```python
from build123d import *

# Parameters (mm, degrees)
SKETCH_1_R          = 0.9
EXTRUDE_1_DEPTH     = 1.8
SKETCH_2_R          = 1.5
EXTRUDE_2_DEPTH     = 1.5
SKETCH_2_3_W        = 1.1
SKETCH_2_3_H        = 0.4
CUT_EXTRUDE_1_DEPTH = 11.647300127


with BuildPart() as part:
    # Sketch 1 → Extrude 1 (new body)
    with BuildSketch(Plane.XY):
        with BuildLine():
            Line((-2.839013913, -0.25), (-6.05, -0.25))
            Line((-6.05, -0.25), (-6.05, -1.65))
            Line((-6.05, -1.65), (-7.95, -1.65))
            Line((-7.95, -1.65), (-7.95, -3.35))
            Line((-7.95, -3.35), (-6.05, -3.35))
            Line((-6.05, -3.35), (-6.05, -5.95))
            ThreePointArc((-6.05, -5.95), (-5.15, -5.05), (-4.25, -5.95))
            ThreePointArc((-4.25, -5.95), (-4.513603897, -6.586396103), (-5.15, -6.85))
            Line((-5.15, -6.85), (4.65, -6.85))
            Line((4.65, -6.85), (4.65, -5.95))
            Line((4.65, -5.95), (6.55, -5.95))
            Line((6.55, -5.95), (6.55, -4.25))
            Line((6.55, -4.25), (4.65, -4.25))
            Line((4.65, -4.25), (4.65, -2.85))
            Line((4.65, -2.85), (0, -2.85))
            ThreePointArc((0, -2.85), (-1.924837655, -2.101784956), (-2.839013913, -0.25))
        make_face()
        with Locations((-5.15, -5.95)):
            Circle(SKETCH_1_R)
    extrude(amount=EXTRUDE_1_DEPTH)

    # Sketch 2 → Extrude 2 (add)
    with BuildSketch(Plane(origin=(0, 0, 0), x_dir=(-1, 0, 0), z_dir=(0, 0, -1))):
        with Locations(Location((-2.54, -5.01, 0), (0, 0, 180))):
            Circle(SKETCH_2_R)
        with Locations(Location((3.81, -2.54, 0), (0, 0, 180))):
            Circle(SKETCH_2_R)
    extrude(amount=EXTRUDE_2_DEPTH)

    # Sketch 2_3 → Cut-Extrude 1 (cut, through all)
    with BuildSketch(Plane(origin=(0, 0, 0), x_dir=(-1, 0, 0), z_dir=(0, 0, -1))):
        with Locations((-2.54, -5.01)):
            Rectangle(SKETCH_2_3_W, SKETCH_2_3_H)
        with Locations((3.81, -2.54)):
            Rectangle(SKETCH_2_3_W, SKETCH_2_3_H)
    extrude(amount=-CUT_EXTRUDE_1_DEPTH, mode=Mode.SUBTRACT)


solid = part.part
```
Here's how the part is built. I have some questions about the finished solid (model axes, mm). A direction names the side the tool comes from. Coordinates: 2 decimals unless noted, no trailing zeros. Write each loop counter-clockwise with the first axis right and the second up, starting at its lowest first coordinate (ties: lowest second). Pieces come first, ordered by that corner, then holes. Notation, with made-up numbers: (83, 59) -> (106, 59) arc R26 cw to (106, 75) -> close; hole circle Ø6 at (87, 22). An arc over 180 degrees is marked (long way). Use a Markdown table: item, result. Add a question column.
(1) If we section it at B-B, the plane y = -5.01: Write out the boundary of the cut face in (x, z).
(2) I'm going to push flat-ended pins straight in: P1, Ø0.5, axis at x = 1.5, z = 1, coming from the +Y side; P2, Ø2, axis at x = -1, y = -4.5, coming from the -Z side; P3, Ø0.9, axis at x = 6, z = 0.5, coming from the +Y side. Where does each tip first touch, or does it pass through?
(3) Please list where these lines run through material, in increasing order: line 1 (Y direction, x = 2.25, z = 0.15); line 2 (Y direction, x = -4.25, z = 0.25); line 3 (Z direction, x = 0.75, y = -6.5).
(4) We'd pull the mould along X, two halves only. Please class faces 5 (the flat face through (2.5, -4.81, 0.9)), 6 (the flat face through (2, -2.85, 1)), 7 (the flat face through (-6.05, -5, 1)): +X half, -X half, draft (parallel to the pull), parting line (faces both ways), or undercut.
(5) If we section it at D-D, the plane z = -0.9: Write out the boundary of the cut face in (x, y), and give its area (3 significant figures).
(6) If we section it at A-A, the plane z = 0.95: Write out the boundary of the cut face in (x, y).
(7) If we section it at C-C, the plane x = 2.54: Write out the boundary of the cut face in (y, z).
(8) For faces 1 (the cylindrical face through (3.23, -3.68, -0.74)), 2 (the flat face through (4.65, -6.4, 0.9)), 3 (the flat face through (6, -4.25, 1)), 4 (the flat face through (-7, -1.65, 1)), which set-ups out of +Z, -Z, +X, -X, +Y, -Y let a thin tool reach every point of the face, with its end or its side?
Outcome:
| question | item | result |
|---|---|---|
| 1 | outline | (-6.05, 0) -> (1.04, 0) -> (1.04, -1.5) -> (4.04, -1.5) -> (4.04, 0) -> (6.55, 0) -> (6.55, 1.8) -> (3.09, 1.8) -> (3.09, 0) -> (1.99, 0) -> (1.99, 1.8) -> (-6.05, 1.8) -> close |
| 2 | P1 | stops at y = -2.85 |
| 2 | P2 | stops at z = 0 |
| 2 | P3 | stops at y = -4.25 |
| 3 | line 1 | y = -6.85 to -5.21, -4.81 to -2.85 |
| 3 | line 2 | y = -6.85 to -2.74, -2.34 to -0.25 |
| 3 | line 3 | z = 0 to 1.8 |
| 4 | face 5 | undercut |
| 4 | face 6 | draft |
| 4 | face 7 | -X half |
| 5 | outline | circle Ø3 at (-3.81, -2.54); circle Ø3 at (2.54, -5.01) |
| 5 | area | 14.1 mm^2 |
| 6 | outline | (-7.95, -3.35) -> (-6.05, -3.35) -> (-6.05, -5.95) arc R0.9 ccw to (-5.15, -6.85) -> (4.65, -6.85) -> (4.65, -5.95) -> (6.55, -5.95) -> (6.55, -4.25) -> (4.65, -4.25) -> (4.65, -2.85) -> (0, -2.85) arc R2.85 cw to (-2.84, -0.25) -> (-6.05, -0.25) -> (-6.05, -1.65) -> (-7.95, -1.65) -> close; hole (-4.36, -2.74) -> (-3.26, -2.74) -> (-3.26, -2.34) -> (-4.36, -2.34) -> close; hole (1.99, -5.21) -> (3.09, -5.21) -> (3.09, -4.81) -> (1.99, -4.81) -> close |
| 7 | outline | (-6.85, 0) -> (-6.51, 0) -> (-6.51, -1.5) -> (-3.51, -1.5) -> (-3.51, 0) -> (-2.85, 0) -> (-2.85, 1.8) -> (-4.81, 1.8) -> (-4.81, 0) -> (-5.21, 0) -> (-5.21, 1.8) -> (-6.85, 1.8) -> close |
| 8 | face 1 | -Z |
| 8 | face 2 | +Z, -Z, +X, -Y |
| 8 | face 3 | +Z, -Z, +X, +Y |
| 8 | face 4 | +Z, -Z, -X, +Y |
